For this review, take the finished solid that the model builds, in its own axes (mm). A direction names the side the tool comes from. Give positions to 0.01 mm unless a question says otherwise; leave off trailing zeros. Order: outer loops, then holes, each group sorted by start corner. A loop starts at its lowest first (then second) coordinate and runs counter-clockwise, first axis right, second up. Notation, with made-up numbers: M 31,3.5 L 41,3.5 A17 cw 41,10.5 Z; hole C 40,50 d2. An arc over 180 degrees is marked long. Answer as CSV lines item,"result". Start each with the question number.
1. Machinability: for faces 1 (the flat face through (-22.21, -9.51, -3.76)), 2 (the flat face through (12.192, -10, -18)), 3 (the flat face through (20, 6.096, -4)), which of the approach directions +Z, -Z, +X, -X, +Y, -Y give a long, thin tool a straight path to every point of the face, cutting with its end or side? Answer none if there is none.
2. Mouldability with a two-part tool opening along Y and no side actions: class faces 4 (the flat face through (13, 0, 13.945)), 5 (the cylindrical face through (16.4, 7.11, 7.9)), 6 (the flat face through (0, 0, 0)) as pulls with the +Y half, pulls with the -Y half, needs draft (parallel to the pull), parting line crosses it, or undercut.
3. We need section C-C, the plane x = 16. Give the boundary of the cut face in (y, z).
4. Clearance check with flat-ended pins moving along their axes: P1, Ø0.5, axis at x = 0, y = -14.5, coming from the -Z side; P2, Ø13.5, axis at x = -14, y = -0.5, coming from the +Z side; P3, Ø5, axis at x = -11.5, z = -21, coming from the +Y side; P4, Ø1.2, axis at y = -10, z = -20, coming from the +X side. State where each tip first meets the part, or that it passes through.
5. We need section A-A, the plane y = 0. Give the boundary of the cut face in (x, z), and give its area (3 significant figures).
6. We need section D-D, the plane z = -20. Give the boundary of the cut face in (x, y), and give its area (3 significant figures).
7. For line 1 along Y through (x, z) = (0, -8.15); line 2 along Z through (x, y) = (-17, 3.75); line 3 along Z through (x, y) = (-6.5, 2.5), list the stretches that pass through material, from the lowest coordinate up.
8. We need section B-B, the plane z = -1. Give the boundary of the cut face in (x, y), and give its area (3 significant figures).
Autodesk Inventor part; units mm, degrees
ref_plane "Work Plane1" through (-22.86, -10.668, 1.778) normal (0, -1, 0) x (1, 0, 0)
ref_plane "YZ Plane" through (0, 0, 0) normal (1, 0, 0) x (0, 1, 0)
ref_plane "XZ Plane" through (0, 0, 0) normal (0, 1, 0) x (-1, 0, 0)
sketch "Sketch1" plane through (0, 0, 0) normal (0, 0, 1) x (1, 0, 0)
  line L0 (-22.86, 10.668) -> (22.86, 10.668)
  line L1 (22.86, 10.668) -> (22.86, -10.668)
  line L2 (22.86, -10.668) -> (-22.86, -10.668)
  line L3 (-22.86, -10.668) -> (-22.86, 10.668)
  point P0 (0, 0)
  point P1 (-22.86, 0)
  point P2 (0, 10.668)
  dimension "d0" = 45.72
  dimension "d1" = 21.336
extrude "Extrusion1" add sketch "Sketch1" along normal blind 1.778
sketch "Sketch2" plane through (0, 0, 1.778) normal (0, 0, 1) x (1, 0, 0)
  circle A0 centre (-12.7, 0) radius 8.0137
  circle A1 centre (12.7, 0) radius 8.0137
  point P0 (0, 0)
  dimension "d4" = 16.0274
  dimension "d5" = 16.0274
  dimension "d6" = 12.7
  dimension "d7" = 12.7
extrude "Extrusion2" add sketch "Sketch2" along normal blind 12.4206
sketch "Sketch3" plane through (-12.7, 0, 14.1986) normal (0, 0, 1) x (1, 0, 0)
  circle A0 centre (0, 0) radius 8.0137
  circle A1 centre (25.4, 0) radius 8.0137
  circle A2 centre (0, 0) radius 6.2357
  circle A3 centre (25.4, 0) radius 6.2357
  point P0 (12.7, 0)
  dimension "d11" = 1.778
  dimension "d12" = 1.778
extrude "Extrusion3" cut sketch "Sketch3" against normal blind 0.254 contours A2 | A3
sketch "Sketch4" plane through (0, 0, 0) normal (0, 0, -1) x (-1, 0, 0)
  line L0 (-18.9005, 6.096) -> (-21.5402, 6.096)
  line L1 (-21.5402, 6.096) -> (-22.86, 8.382)
  line L2 (-22.86, 8.382) -> (-21.5402, 10.668)
  line L3 (-21.5402, 10.668) -> (-18.9005, 10.668)
  line L4 (-18.9005, 10.668) -> (-17.5807, 8.382)
  line L5 (-17.5807, 8.382) -> (-18.9005, 6.096)
  line L6 (21.5402, -10.668) -> (18.9005, -10.668)
  line L7 (18.9005, -10.668) -> (17.5807, -8.382)
  line L8 (17.5807, -8.382) -> (18.9005, -6.096)
  line L9 (18.9005, -6.096) -> (21.5402, -6.096)
  line L10 (21.5402, -6.096) -> (22.86, -8.382)
  line L11 (22.86, -8.382) -> (21.5402, -10.668)
  line L12 (22.86, 10.668) -> (-22.86, 10.668)
  line L13 (-22.86, -10.668) -> (22.86, -10.668)
  line L14 (22.86, -10.668) -> (22.86, 10.668)
  line L15 (-22.86, 10.668) -> (-22.86, -10.668)
  point P0 (0, 0)
  point P1 (-20.2204, 8.382)
  point P2 (20.2204, -8.382)
  dimension "d15" = 4.572
  dimension "d16" = 4.572
extrude "Extrusion4" add sketch "Sketch4" along normal blind 7.62 contours L0 L1 L2 L3 L4 L5 | L7 L8 L9 L10 L11 L6
sketch "Sketch5" plane through (0, 0, -7.62) normal (0, 0, -1) x (-1, 0, 0)
  line L0 (18.9005, -10.668) -> (17.5807, -8.382)
  line L1 (17.5807, -8.382) -> (18.9005, -6.096)
  line L2 (18.9005, -6.096) -> (21.5402, -6.096)
  line L3 (21.5402, -6.096) -> (22.86, -8.382)
  line L4 (22.86, -8.382) -> (22.86, 10.668)
  line L5 (22.86, 10.668) -> (-18.9005, 10.668)
  line L6 (-18.9005, 10.668) -> (-17.5807, 8.382)
  line L7 (-17.5807, 8.382) -> (-18.9005, 6.096)
  line L8 (-18.9005, 6.096) -> (-21.5402, 6.096)
  line L9 (-21.5402, 6.096) -> (-22.86, 8.382)
  line L10 (-22.86, 8.382) -> (-22.86, -10.668)
  line L11 (-22.86, -10.668) -> (18.9005, -10.668)
  line L12 (-21.5402, 10.668) -> (-22.86, 10.668)
  line L13 (-22.86, 10.668) -> (-22.86, 8.382)
  line L14 (-18.9005, 10.668) -> (-21.5402, 10.668)
  line L15 (18.9005, -10.668) -> (21.5402, -10.668)
  line L16 (22.86, -10.668) -> (22.86, -8.382)
  line L17 (21.5402, -10.668) -> (22.86, -10.668)
  line L18 (-21.5402, 6.096) -> (-18.9005, 6.096)
  line L19 (-22.86, 8.382) -> (-21.5402, 6.096)
  line L20 (-22.86, 10.668) -> (22.86, 10.668)
  line L21 (-22.86, 10.668) -> (22.86, 10.668)
  line L22 (22.86, 10.668) -> (22.86, -10.668)
  line L23 (22.86, -10.668) -> (-22.86, -10.668)
  line L24 (-22.86, -10.668) -> (-22.86, 10.668)
  point P0 (0, 0)
extrude "Extrusion5" add sketch "Sketch5" along normal blind 1.524
ref_plane "Work Plane1" through (-22.86, -10.668, 1.778) normal (0, -1, 0) x (1, 0, 0)
sketch "Sketch6" plane through (-22.86, -10.668, 1.778) normal (0, -1, 0) x (1, 0, 0)
  line L0 (0, -1.778) -> (0, -9.398)
  line L1 (22.352, -10.922) -> (22.352, -27.305) construction
  line L2 (35.052, -10.922) -> (35.052, -27.305)
  line L3 (9.652, -27.305) -> (9.652, -10.922)
  arc A0 (9.652, -27.305) -> (35.052, -27.305) centre (22.352, -27.305) ccw
  line L4 (0, -10.922) -> (45.72, -10.922)
  line L5 (35.052, -10.922) -> (9.652, -10.922)
  point P0 (22.86, -1.778)
  point P1 (22.352, -19.1135)
  point P2 (22.352, -40.005)
  dimension "d23" = 9.652
  dimension "d25" = 25.4
  dimension "d26" = 29.083
  dimension "d27" = 0
  dimension "d28" = 0
extrude "Extrusion6" add sketch "Sketch6" against normal blind 1.524
fillet "Fillet1" radius 0.9525 1 edges at (-0.508, -9.144, -9.144)
sketch "Sketch7" plane through (0, 0, -9.144) normal (0, 0, -1) x (-1, 0, 0)
  circle A0 centre (0, 0) radius 5.7785
  dimension "d32" = 11.557
extrude "Extrusion7" cut sketch "Sketch7" against normal up to next
sketch "Sketch8" plane through (-22.86, -10.668, 1.778) normal (0, -1, 0) x (1, 0, 0)
  arc A0 (9.652, -27.305) -> (35.052, -27.305) centre (22.352, -27.305) ccw
  line L0 (9.652, -27.305) -> (9.652, -10.922)
  line L1 (35.052, -10.922) -> (35.052, -27.305)
  circle A1 centre (22.352, -27.305) radius 4.0005
  circle A2 centre (22.352, -35.6362) radius 1.2065
  circle A3 centre (30.6832, -27.305) radius 1.2065
  circle A4 centre (14.0208, -27.305) radius 1.2065
  circle A5 centre (22.352, -18.9738) radius 1.2065
  point P0 (22.86, -1.778)
  dimension "d35" = 8.001
  dimension "d36" = 2.413
  dimension "d37" = 2.413
  dimension "d38" = 2.413
  dimension "d39" = 2.413
  dimension "d40" = 8.3312
  dimension "d41" = 8.3312
  dimension "d42" = 8.3312
  dimension "d43" = 8.3312
extrude "Extrusion8" cut sketch "Sketch8" against normal through all
fillet "Fillet2" radius 1.27 2 edges at (12.192, -9.4298, -9.144) (-13.208, -9.4298, -9.144)
sketch "Sketch9" plane through (0, 0, 1.778) normal (0, 0, 1) x (1, 0, 0)
  line L0 (-3.4317, -16.51) -> (-2.7967, -16.51)
  line L1 (-2.7967, -16.51) -> (-2.7967, -8.128)
  line L2 (-2.7967, -8.128) -> (-3.4317, -8.128)
  line L3 (-3.4317, -8.128) -> (-3.4317, -16.51)
  line L4 (-0.3175, -16.51) -> (0.3175, -16.51)
  line L5 (0.3175, -16.51) -> (0.3175, -8.128)
  line L6 (0.3175, -8.128) -> (-0.3175, -8.128)
  line L7 (-0.3175, -8.128) -> (-0.3175, -16.51)
  line L8 (2.7967, -16.51) -> (3.4317, -16.51)
  line L9 (3.4317, -16.51) -> (3.4317, -8.128)
  line L10 (3.4317, -8.128) -> (2.7967, -8.128)
  line L11 (2.7967, -8.128) -> (2.7967, -16.51)
  line L12 (-22.86, -10.668) -> (22.86, -10.668)
  point P0 (0, 0)
  point P1 (0, -8.128)
  point P2 (-2.7967, -12.319)
  point P3 (-0.3175, -12.319)
  point P4 (2.7967, -12.319)
  point P5 (-3.1142, -8.128)
  dimension "d47" = 2.4792
  dimension "d48" = 2.4792
  dimension "d49" = 0.635
  dimension "d50" = 8.382
  dimension "d51" = 2.54
extrude "Extrusion9" add sketch "Sketch9" along normal blind 0.635
equation "\"d5\" = d4"
equation "\"d12\" = d11"
equation "\"d16\" = d15"
equation "\"d37\" = d36"
equation "\"d38\" = d36"
equation "\"d39\" = d36"
equation "\"d41\" = d40"
equation "\"d42\" = d40"
equation "\"d43\" = d40"
equation "\"d48\" = d47"
properties part number "Ultrasound"
Result set:
1,face 1,"-X, -Y"
1,face 2,"-Z, +X, +Y, -Y"
1,face 3,"+X, -X, -Y"
2,face 4,"undercut"
2,face 5,"parting line crosses it"
2,face 6,"needs draft"
3,outline,"M -10.67,-9.14 L 10.67,-9.14 L 10.67,-7.62 L -10.67,-7.62 Z; M -10.67,0 L 10.67,0 L 10.67,1.78 L 7.3,1.78 L 7.3,14.2 L 5.29,14.2 L 5.29,13.94 L -5.29,13.94 L -5.29,14.2 L -7.3,14.2 L -7.3,1.78 L -10.67,1.78 Z"
4,P1,"z = 1.78"
4,P2,"z = 14.2"
4,P3,"y = -9.14"
4,P4,"x = 12.19"
5,outline,"M -22.86,-9.14 L -5.78,-9.14 L -5.78,-7.62 L -22.86,-7.62 Z; M -22.86,0 L 22.86,0 L 22.86,1.78 L 20.71,1.78 L 20.71,14.2 L 18.94,14.2 L 18.94,13.94 L 6.46,13.94 L 6.46,14.2 L 4.69,14.2 L 4.69,1.78 L -4.69,1.78 L -4.69,14.2 L -6.46,14.2 L -6.46,13.94 L -18.94,13.94 L -18.94,14.2 L -20.71,14.2 L -20.71,1.78 L -22.86,1.78 Z; M 5.78,-9.14 L 22.86,-9.14 L 22.86,-7.62 L 5.78,-7.62 Z"
5,area,"525 mm2"
6,outline,"M -13.21,-10.67 L 12.19,-10.67 L 12.19,-9.14 L -13.21,-9.14 Z"
6,area,"38.7 mm2"
7,line 1,"-10.67 to -5.78, 5.78 to 10.67"
7,line 2,"-9.14 to -7.62, 0 to 13.94"
7,line 3,"-9.14 to -7.62, 0 to 14.2"
8,outline,"M -22.86,-8.38 L -21.54,-10.67 L -18.9,-10.67 L -17.58,-8.38 L -18.9,-6.1 L -21.54,-6.1 Z; M 17.58,8.38 L 18.9,6.1 L 21.54,6.1 L 22.86,8.38 L 21.54,10.67 L 18.9,10.67 Z"
8,area,"36.2 mm2"
